Verification items for this drawing (mm, ordinates from the low corner). A direction names the side the tool comes from. Round coordinates to 2 decimals unless told otherwise and drop trailing zeros. Order: outer loops, then holes, each group sorted by start corner. A loop starts at its lowest first (then second) coordinate and runs counter-clockwise, first axis right, second up. Notation, with made-up numbers: M 44,40.25 L 53,40.25 A16 cw 53,55.25 Z; hole C 47.25,85 d6. An arc over 180 degrees is marked long. Return JSON: item names as keys, results as strings. Group by question number.
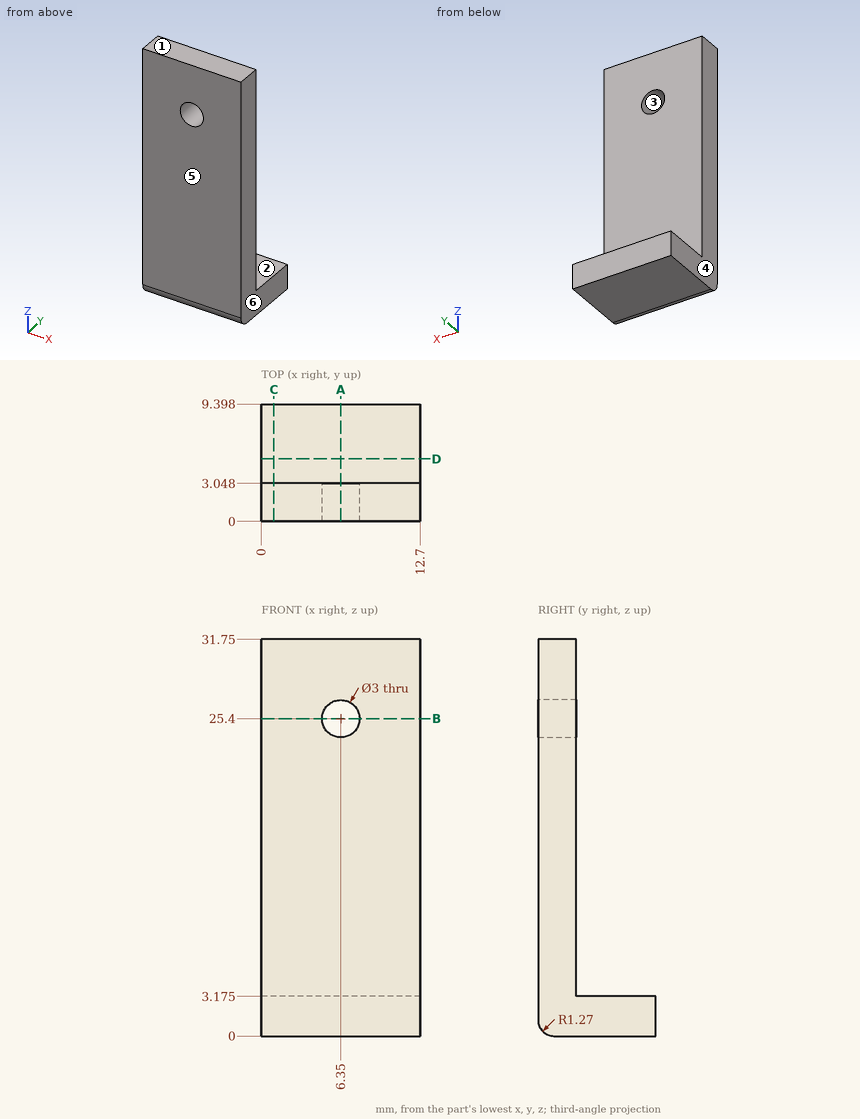
1. Cross-section at B-B (z = 25.4). Enter the section's corners in (x, y), plus the area to 3 significant figures.
2. Access from +Z, -Z, +X, -X, +Y, -Y to the whole of each face (thin tool, end or side, straight path). Record for the marked faces 1 and 2.
3. Cross-section at C-C (x = 1). Enter the section's corners in (y, z) (3 decimals).
4. Cross-section at D-D (y = 5). Enter the section's corners in (x, z) (3 decimals).
5. Draft check along X on the marked faces 3, 4, 5 and 6. Enter one of: +X half, -X half, draft (parallel to the pull), parting line (faces both ways), or undercut.
6. Cross-section at A-A (x = 6.35). Enter the section's corners in (y, z) (3 decimals).
7. Thickness scan on line 1 along X through (y, z) = (1.7, 25.4); line 2 along Y through (x, z) = (12.25, 13.5); line 3 along Z through (x, y) = (10.5, 7.75) (3 decimals). Record the ranges inside material, lowest first. Write a range as from..to.
8. Go/stop test with flat-tipped pins: pin 1 (4 mm diameter, centred on x = 7, z = 24.5, fed in from +Y); pin 2 (3 mm diameter, centred on x = 6, y = 7, fed in from +Z) (3 decimals). Record where each tip stops, or that it passes through.
Computed:
{
 "1": {"outline": "M 0,0 L 4.85,0 L 4.85,3.05 L 0,3.05 Z; M 7.85,0 L 12.7,0 L 12.7,3.05 L 7.85,3.05 Z", "area": "29.6 mm²"},
 "2": {"face 1": "+Z, +X, -X, +Y, -Y", "face 2": "+Z, +X, -X, +Y"},
 "3": {"outline": "M 0,1.27 A1.27 ccw 1.27,0 L 9.398,0 L 9.398,3.175 L 3.048,3.175 L 3.048,31.75 L 0,31.75 Z"},
 "4": {"outline": "M 0,0 L 12.7,0 L 12.7,3.175 L 0,3.175 Z"},
 "5": {"face 3": "undercut", "face 4": "-X half", "face 5": "draft", "face 6": "+X half"},
 "6": {"outline": "M 0,1.27 A1.27 ccw 1.27,0 L 9.398,0 L 9.398,3.175 L 3.048,3.175 L 3.048,23.9 L 0,23.9 Z; M 0,26.9 L 3.048,26.9 L 3.048,31.75 L 0,31.75 Z"},
 "7": {"line 1": "x = 0..4.85, 7.85..12.7", "line 2": "y = 0..3.05", "line 3": "z = 0..3.175"},
 "8": {"pin 1": "stops at y = 3.05", "pin 2": "stops at z = 3.175"}
}
